Answer from the drawing. Dimensions are ordinates in mm from the lowest x, y and z of the part. Give positions to 0.01 mm unless a question says otherwise; leave off trailing zeros. Write each loop counter-clockwise with the first axis right and the second up, starting at its lowest first coordinate (ties: lowest second). Pieces come first, ordered by that corner, then holes. Notation, with made-up numbers: (46, 43) -> (68, 43) arc R12 ccw to (68, 61) -> close; hole circle Ø3 at (83, -18.75). An arc over 180 degrees is marked (long way). Use a Markdown table: item, result. Add a question column.
Q1. Section A-A, the plane x = 243 is taken. Give the vertices of the cut face in (y, z), plus the area to 3 significant figures.
Q2. Consider line 1 (Y direction, x = 186, z = 8); line 2 (X direction, y = 75, z = 11.5); line 3 (Y direction, x = 243, z = 6.5). Determine where each line is inside the solid, lowest interval first.
Q3. For a pull along X with two mould halves and no side action, classify the marked faces 1, 2, 3 and 4 as pulls with the +X half, pulls with the -X half, needs draft (parallel to the pull), parting line crosses it, or undercut.
Q4. Section D-D, the plane x = 138 is taken. Give the vertices of the cut face in (y, z), plus the area to 3 significant figures.
Q5. Section C-C, the plane z = 17.25 is taken. State how many separate pieces and enclosed holes the cut face has, plus the area to 3 significant figures.
Q6. Section B-B, the plane y = 75 is taken. Give the vertices of the cut face in (x, z), plus the area to 3 significant figures.
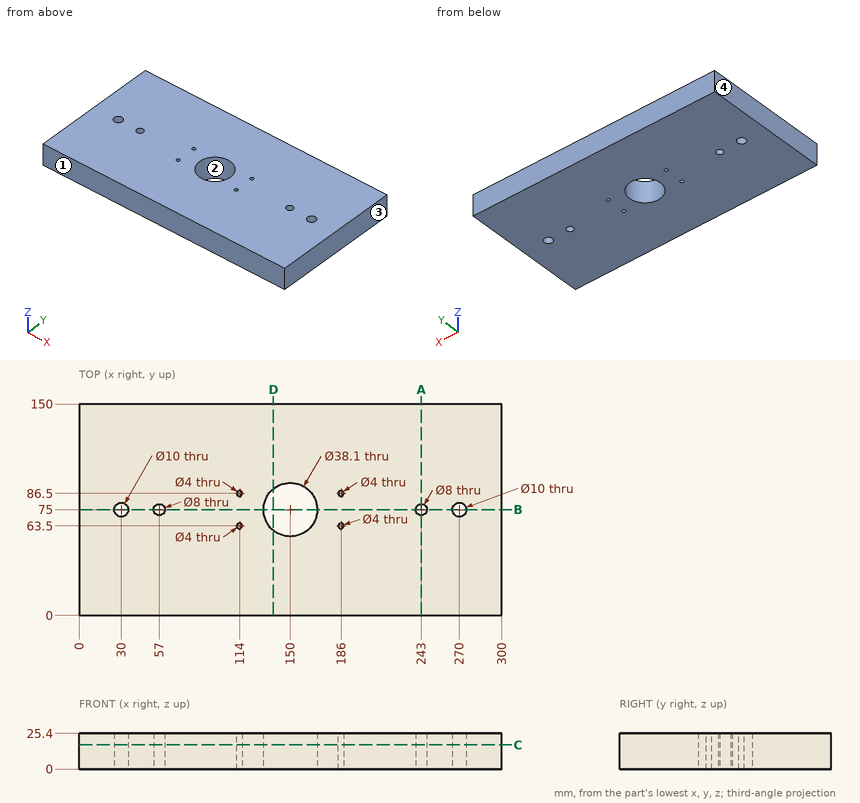
Result set:
| question | item | result |
|---|---|---|
| 1 | outline | (0, 0) -> (71, 0) -> (71, 25.4) -> (0, 25.4) -> close; (79, 0) -> (150, 0) -> (150, 25.4) -> (79, 25.4) -> close |
| 1 | area | 3,610 mm2 |
| 2 | line 1 | y = 0 to 61.5, 65.5 to 84.5, 88.5 to 150 |
| 2 | line 2 | x = 0 to 25, 35 to 53, 61 to 130.95, 169.05 to 239, 247 to 265, 275 to 300 |
| 2 | line 3 | y = 0 to 71, 79 to 150 |
| 3 | face 1 | needs draft |
| 3 | face 2 | undercut |
| 3 | face 3 | pulls with the +X half |
| 3 | face 4 | pulls with the -X half |
| 4 | outline | (0, 0) -> (60.2, 0) -> (60.2, 25.4) -> (0, 25.4) -> close; (89.8, 0) -> (150, 0) -> (150, 25.4) -> (89.8, 25.4) -> close |
| 4 | area | 3,060 mm2 |
| 5 | separate pieces | 1 |
| 5 | enclosed holes | 9 |
| 5 | area | 43,600 mm2 |
| 6 | outline | (0, 0) -> (25, 0) -> (25, 25.4) -> (0, 25.4) -> close; (35, 0) -> (53, 0) -> (53, 25.4) -> (35, 25.4) -> close; (61, 0) -> (130.95, 0) -> (130.95, 25.4) -> (61, 25.4) -> close; (169.05, 0) -> (239, 0) -> (239, 25.4) -> (169.05, 25.4) -> close; (247, 0) -> (265, 0) -> (265, 25.4) -> (247, 25.4) -> close; (275, 0) -> (300, 0) -> (300, 25.4) -> (275, 25.4) -> close |
| 6 | area | 5,740 mm2 |
